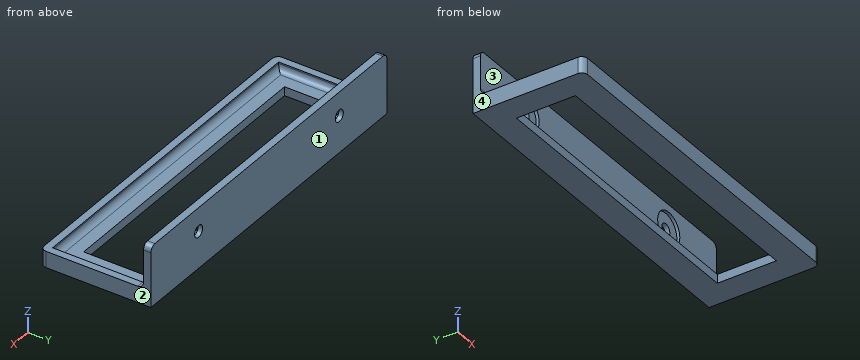
```python
from build123d import *

# Parameters (mm, degrees)
F0_W     = 149.225
F0_H     = 47.625
F0_W_2   = 127
F0_H_2   = 25.4
F1_DEPTH = 3.81
F2_W     = 149.225
F2_H     = 47.625
F2_W_2   = 142.875
F2_H_2   = 41.275
F3_DEPTH = 3.175
F5_DEPTH = 19.05
F6_R     = 2.54
F7_DEPTH = 25.4
F6_R_2   = 6.985
F8_DEPTH = 1.27
F9_R     = 2.54


with BuildPart() as f1:
    # F0 (on Top) → F1 (new body)
    with BuildSketch(Plane.XY):
        Rectangle(F0_W, F0_H)
        Rectangle(F0_W_2, F0_H_2, mode=Mode.SUBTRACT)
    extrude(amount=F1_DEPTH)

    # F2 (on face) → F3 (join)
    with BuildSketch(Plane.XY.offset(3.81)):
        Rectangle(F2_W, F2_H)
        Rectangle(F2_W_2, F2_H_2, mode=Mode.SUBTRACT)
    extrude(amount=F3_DEPTH)

    # F4 (on face) → F5 (join)
    with BuildSketch(Plane.XY.offset(6.985)):
        Polygon((74.6125, 23.8125), (-74.6125, 23.8125), (-74.6125, 20.6375), (-71.4375, 20.6375), (71.4375, 20.6375), (74.6125, 20.6375), align=None)
    extrude(amount=F5_DEPTH)

    # F6 (on face) → F7 (cut)
    with BuildSketch(Plane.XZ.offset(-20.6375)):
        with Locations((-44.45, 15.875)):
            Circle(F6_R)
        with Locations((44.45, 15.875)):
            Circle(F6_R)
    extrude(amount=-F7_DEPTH, mode=Mode.SUBTRACT)

    # F6 (on face) → F8 (cut)
    with BuildSketch(Plane.XZ.offset(-20.6375)):
        with Locations((-44.45, 15.875)):
            Circle(F6_R_2)
        with Locations((-44.45, 15.875)):
            Circle(F6_R, mode=Mode.SUBTRACT)
        with Locations((44.45, 15.875)):
            Circle(F6_R_2)
        with Locations((44.45, 15.875)):
            Circle(F6_R, mode=Mode.SUBTRACT)
    extrude(amount=-F8_DEPTH, mode=Mode.SUBTRACT)

    # F9
    f9_edges = [f1.edges().sort_by_distance(p)[0] for p in [
        (-73.025, 20.6375, 6.985),
        (73.025, 20.6375, 6.985),
        (0, 20.6375, 3.81),
        (74.6125, 22.225, 26.035),
        (-74.6125, 22.225, 26.035),
        (-74.6125, -23.8125, 3.4925),
        (74.6125, -23.8125, 3.4925),
        (71.4375, 0, 3.81),
        (-71.4375, 0, 3.81),
        (0, -20.6375, 3.81),
    ]]
    fillet(f9_edges, radius=F9_R)


solid = f1.part
```
Geometry: final body of the model. Coordinates: model frame, mm. Face numbers are marked on the shaded views. Coordinates: 2 decimals unless noted, no trailing zeros. Write each question's results on one line, items separated by ' | '.
(1) Mould query, pull axis X, two halves, no side actions, for the marked faces 1, 2, 3 and 4. Classes: +X half, -X half, draft (parallel to the pull), parting line (faces both ways), or undercut.
Values found:
face 1: draft | face 2: +X half | face 3: undercut | face 4: -X half
(2) First-contact query: pin 1 Ø11 at (x, y) = (16.5, 8) entering from +Z; pin 2 Ø1.5 at (x, z) = (-25.5, 13.5) entering from -Y; pin 3 Ø8 at (x, z) = (44.45, 15.875) entering from -Y. Flat tips, straight axial feed; report the tip coordinate or a pass-through.
Values found:
pin 1: stops at z = 3.81 | pin 2: stops at y = 20.64 | pin 3: stops at y = 21.91
(3) Line query: line 1 (Z direction, x = 44.45, y = 22.45) (3 decimals); line 2 (X direction, y = -20.5, z = 6); line 3 (Y direction, x = -4, z = 3.5). Output: solid intervals per line, ascending. Write a range as [from, to].
Values found:
line 1: z = [0, 13.335], [18.415, 26.035] | line 2: x = [-74.61, -71.41], [71.41, 74.61] | line 3: y = [-23.81, -12.7], [12.7, 23.81]
(4) Section query B-B, the plane x = 44.45. Count the separate pieces of the cut face and the enclosed holes in it, plus the area to 3 significant figures.
Values found:
separate pieces: 3 | enclosed holes: 0 | area: 141 mm²
